Work out the finished part from the listing and answer in its coordinate system (mm). Coordinates: 2 decimals unless noted, no trailing zeros. Order: outer loops, then holes, each group sorted by start corner. A loop starts at its lowest first (then second) coordinate and runs counter-clockwise, first axis right, second up. Notation, with made-up numbers: (84, 66.5) - (137, 66.5) arc R35 ccw to (137, 105.5) - close; hole circle Ø8 at (-38.5, 64). An arc over 180 degrees is marked (long way). Answer as a JSON object with one key per item and string values. Group by question number.
1) Find the intervals of material crossed by line 1 along Z through (x, y) = (0, 1.25); line 2 along X through (y, z) = (0.1, 13.5); line 3 along X through (y, z) = (0.95, 9.5), in increasing order.
2) Each of these flat-tipped pins is pushed along its axis until it touches: P1, Ø0.8, axis at y = 1, z = 17.5, coming from the +X side; P2, Ø0.8, axis at x = 11, y = 1, coming from the +Z side. Where does it stop, or does it pass through?
3) Section A-A (y = 0.75) is taken. Count the separate pieces of the cut face and the enclosed holes in it, plus the area to 3 significant figures.
4) Section B-B (z = 16) is taken. Give the vertices of the cut face in (x, y).
5) Section D-D (z = 1.5) is taken. Give the vertices of the cut face in (x, y), plus the area to 3 significant figures.
6) Section C-C (x = 16) is taken. Give the vertices of the cut face in (y, z).
Autodesk Inventor part; units mm, degrees
ref_plane "YZ Plane" through (0, 0, 0) normal (1, 0, 0) x (0, 1, 0)
ref_plane "XZ Plane" through (0, 0, 0) normal (0, 1, 0) x (-1, 0, 0)
ref_plane "XY Plane" through (0, 0, 0) normal (0, 0, 1) x (1, 0, 0)
sketch "main" plane through (0, 0, 0) normal (0, 0, 1) x (1, 0, 0)
  circle A0 centre (19.7324, 21.1672) radius 2.1844
  circle A1 centre (19.7324, -16.9328) radius 2.1844
  circle A2 centre (-18.3676, -16.9328) radius 2.1844
  arc A3 (24.4949, 21.1672) -> (16.3648, 24.5348) centre (19.7324, 21.1672) ccw
  arc A4 (-21.7352, -13.5652) -> (-18.3676, -21.6953) centre (-18.3676, -16.9328) ccw
  arc A5 (19.7324, -21.6953) -> (24.4949, -16.9317) centre (19.7324, -16.9328) ccw
  line L0 (19.7324, -21.6953) -> (-18.3676, -21.6953)
  line L1 (24.4949, 21.1672) -> (24.4949, -16.9317)
  line L2 (16.3648, 24.5348) -> (-21.7352, -13.5652)
  line L3 (13.3824, -12.1703) -> (-3.0373, -12.1703)
  line L4 (-4.1599, -9.4602) -> (12.2599, 6.9595)
  line L5 (14.9699, 5.837) -> (14.9699, -10.5828)
  arc A6 (13.3824, -12.1703) -> (14.9699, -10.5828) centre (13.3824, -10.5828) ccw
  arc A7 (14.9699, 5.837) -> (12.2599, 6.9595) centre (13.3824, 5.837) ccw
  arc A8 (-4.1599, -9.4602) -> (-3.0373, -12.1703) centre (-3.0373, -10.5828) ccw
  circle A9 centre (19.7324, -4.2328) radius 2.1844
  point P0 (6.6792, -3.8964)
  dimension "d0" = 9.525
  dimension "d1" = 9.525
  dimension "d2" = 9.525
  dimension "d5" = 9.525
  dimension "d6" = 1.5875
  dimension "d7" = 1.5875
  dimension "d11" = 4.3688
sketch "Sketch1" plane through (0, 0, 0) normal (0, 1, 0) x (-1, 0, 0)
  circle A0 centre (0, 38.1) radius 2.1844
  circle A1 centre (0, 0) radius 2.1844
  circle A2 centre (-38.1, 0) radius 2.1844
  arc A3 (4.7625, 38.1) -> (-3.3676, 41.4676) centre (0, 38.1) ccw
  arc A4 (-41.4676, 3.3676) -> (-38.1, -4.7625) centre (-38.1, 0) ccw
  arc A5 (0, -4.7625) -> (4.7625, 0.0011) centre (0, 0) ccw
  line L0 (0, -4.7625) -> (-38.1, -4.7625)
  line L1 (4.7625, 38.1) -> (4.7625, 0.0011)
  line L2 (-3.3676, 41.4676) -> (-41.4676, 3.3676)
  line L3 (-6.35, 4.7625) -> (-22.7697, 4.7625)
  line L4 (-23.8923, 7.4725) -> (-7.4725, 23.8923)
  line L5 (-4.7625, 22.7697) -> (-4.7625, 6.35)
  arc A6 (-6.35, 4.7625) -> (-4.7625, 6.35) centre (-6.35, 6.35) ccw
  arc A7 (-4.7625, 22.7697) -> (-7.4725, 23.8923) centre (-6.35, 22.7697) ccw
  arc A8 (-23.8923, 7.4725) -> (-22.7697, 4.7625) centre (-22.7697, 6.35) ccw
  circle A9 centre (0, 12.7) radius 2.1844
extrude "Extrusion1" add sketch "Sketch1" along normal blind 1.5875
properties part number "right_angle_gusset" material "Acetal Resin, White"
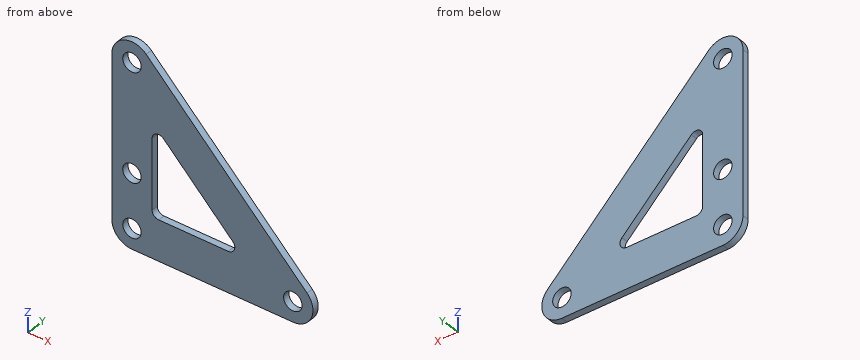
Report:
{
 "1": {"line 1": "z = -4.76 to -2.18, 2.18 to 10.52, 14.88 to 35.92, 40.28 to 42.86", "line 2": "x = -4.76 to -2.03, 2.03 to 4.76, 17.86 to 31.34", "line 3": "x = -4.76 to 4.76, 21.86 to 35.34"},
 "2": {"P1": "stops at x = 27.74", "P2": "stops at z = 34.24"},
 "3": {"separate pieces": "1", "enclosed holes": "5", "area": "1,120 mm²"},
 "4": {"outline": "(-4.76, 0) - (4.76, 0) - (4.76, 1.59) - (-4.76, 1.59) - close; (15.36, 0) - (28.84, 0) - (28.84, 1.59) - (15.36, 1.59) - close"},
 "5": {"outline": "(-4.76, 0) - (-1.59, 0) - (-1.59, 1.59) - (-4.76, 1.59) - close; (1.59, 0) - (36.51, 0) - (36.51, 1.59) - (1.59, 1.59) - close; (39.69, 0) - (42.62, 0) - (42.62, 1.59) - (39.69, 1.59) - close", "area": "65.1 mm²"},
 "6": {"outline": "(0, -4.76) - (1.59, -4.76) - (1.59, 4.76) - (0, 4.76) - close; (0, 15.36) - (1.59, 15.36) - (1.59, 28.84) - (0, 28.84) - close"}
}
